Autodesk Inventor part; units mm, degrees
ref_plane "YZ Plane" through (0, 0, 0) normal (1, 0, 0) x (0, 1, 0)
ref_plane "XZ Plane" through (0, 0, 0) normal (0, 1, 0) x (-1, 0, 0)
ref_plane "XY Plane" through (0, 0, 0) normal (0, 0, 1) x (1, 0, 0)
ref_plane "Work Plane1" through (-14.5039, 0, 0) normal (0, 0, 1) x (1, 0, 0)
sketch "Sketch1" plane through (-14.5039, 0, 0) normal (0, 0, 1) x (1, 0, 0)
  line L0 (-0.3057, 380.2711) -> (-25.3057, 380.2711)
  line L1 (-25.3057, 380.2711) -> (-25.3057, 360.2711)
  line L2 (-25.3057, 360.2711) -> (-0.3057, 360.2711)
  line L3 (-0.3057, 360.2711) -> (-0.3057, 380.2711)
  arc A0 (-39.9465, 315.9933) -> (-39.9465, 424.5488) centre (-105.3057, 370.2711) ccw
  line L4 (-40.5531, 425.2711) -> (-40.5531, 315.2711) construction
  line L5 (-40.5531, 425.2711) -> (69.4469, 425.2711) construction
  line L6 (-41.4851, 315.2711) -> (-42.3392, 315.2711)
  line L7 (-41.4851, 425.2711) -> (-42.3392, 425.2711)
  arc A1 (-43.0983, 316.922) -> (-43.0983, 423.6201) centre (-105.3057, 370.2711) ccw
  arc A2 (-41.4851, 315.2711) -> (-39.9465, 315.9933) centre (-41.4851, 317.2711) ccw
  arc A3 (-39.9465, 424.5488) -> (-41.4851, 425.2711) centre (-41.4851, 423.2711) ccw
  arc A4 (-42.3392, 425.2711) -> (-43.0983, 423.6201) centre (-42.3392, 424.2711) ccw
  arc A5 (-43.0983, 316.922) -> (-42.3392, 315.2711) centre (-42.3392, 316.2711) ccw
  point P0 (14.5039, 0)
  point P1 (-44.5531, 315.2711)
  point P2 (-44.5531, 425.2711)
  point P3 (-20.938, 380.2711)
  point P4 (-20.938, 360.2711)
  dimension "d0" = 25
  dimension "d1" = 20
  dimension "d2" = 110
  dimension "d3" = 90
  dimension "d4" = 45
  dimension "d5" = 105
  dimension "d6" = 4
  dimension "d22" = 2
  dimension "d23" = 2
  dimension "d24" = 1
extrude "Extrusion1" add sketch "Sketch1" along normal blind 165 contours L3 L2 A0 L0 | A0 L2 A1 L0 | L0 A1 A4 L7 A3 A0 | A0 A2 L6 A5 A1 L2
sketch "Sketch2" plane through (-14.8095, 360.2711, 0) normal (1, 0, 0) x (0, 0, -1)
  circle A0 centre (-30, 10) radius 2.75
  circle A1 centre (-135, 10) radius 2.75
  line L0 (-165, 0) -> (-165, 20)
  line L1 (0, 0) -> (0, -44.2778)
  line L2 (-30, 10) -> (-135, 10)
  line L3 (0, -45) -> (-165, -45)
  point P0 (0, -360.2711)
  dimension "d10" = 5.5
  dimension "d11" = 5.5
  dimension "d12" = 30
  dimension "d13" = 30
  dimension "d17" = 55
extrude "Extrusion2" cut sketch "Sketch2" against normal through all
ref_plane "Work Plane2" through (-39.8095, 360.2711, 0) normal (1, 0, 0) x (0, 0, -1)
sketch "Sketch4" plane through (-39.8095, 360.2711, 0) normal (1, 0, 0) x (0, 0, -1)
  circle A0 centre (-30, 10) radius 2.75
  circle A1 centre (-30, 10) radius 5.75
  circle A2 centre (-135, 10) radius 2.75
  circle A3 centre (-135, 10) radius 5.75
  point P0 (0, -360.2711)
  dimension "d18" = 11.5
  dimension "d19" = 11.5
extrude "Extrusion3" cut sketch "Sketch4" along normal blind 20 contours A0 | A1 | A3
equation "\"d4\" = -0.5 * d1 + 0.5 * d2"
properties part number "LegSupport"
Here's how the part is built. I have some questions about the finished solid (model axes, mm). A direction names the side the tool comes from. Give positions to 0.01 mm unless a question says otherwise; leave off trailing zeros. Loops run counter-clockwise (first coordinate to the right, second up) from the corner with the lowest first, then second, coordinate; pieces in that order, holes last. Notation, with made-up numbers: M 86.5,51 L 94.5,51 A5 cw 94.5,60 Z; hole C 6,33.5 d4. An arc over 180 degrees is marked long. Return JSON: item names as keys, results as strings.
Item 1: Imagine slicing it at B-B on z = 52. List the corners of the cut face in (x, y) for me.
A:
{"outline": "M -57.6,316.92 A1 ccw -56.84,315.27 L -55.99,315.27 A2 ccw -54.45,315.99 A84.96 ccw -35.44,360.27 L -14.81,360.27 L -14.81,380.27 L -35.44,380.27 A84.96 ccw -54.45,424.55 A2 ccw -55.99,425.27 L -56.84,425.27 A1 ccw -57.6,423.62 A81.95 cw Z"}
Item 2: Imagine slicing it at D-D on x = -43. List the corners of the cut face in (y, z) for me.
A:
{"outline": "M 333.96,0 L 341.7,0 L 341.7,165 L 333.96,165 Z; M 398.84,0 L 406.58,0 L 406.58,165 L 398.84,165 Z"}
Item 3: Imagine slicing it at C-C on x = -33.5. List the corners of the cut face in (y, z) for me, then the cut area to 3 significant figures.
A:
{"outline": "M 360.27,0 L 380.27,0 L 380.27,165 L 360.27,165 Z; hole C 370.27,30 d11.5; hole C 370.27,135 d11.5", "area": "3,090 mm^2"}
Item 4: Imagine slicing it at A-A on z = 135. List the corners of the cut face in (x, y) for me, then the cut area to 3 significant figures.
A:
{"outline": "M -57.6,316.92 A1 ccw -56.84,315.27 L -55.99,315.27 A2 ccw -54.45,315.99 A84.96 ccw -35.44,360.27 L -14.81,360.27 L -14.81,367.52 L -19.81,367.52 L -19.81,364.52 L -38.06,364.52 A81.95 cw Z; M -57.6,423.62 A81.95 cw -38.06,376.02 L -19.81,376.02 L -19.81,373.02 L -14.81,373.02 L -14.81,380.27 L -35.44,380.27 A84.96 ccw -54.45,424.55 A2 ccw -55.99,425.27 L -56.84,425.27 A1 ccw Z", "area": "528 mm^2"}
Item 5: Thinking about a two-plate mould opening in Z: for faces 1 (the flat face through (-33, 371, 0)), 2 (the cylindrical face through (-41.877, 404.1, 81.345)), 3 (the cylindrical face through (-17.275, 367.586, 30.596)), which applies, released by +Z, released by -Z, zero draft, split by the parting line, or undercut?
A:
{"face 1": "released by -Z", "face 2": "zero draft", "face 3": "undercut"}
Item 6: I'm going to push flat-ended pins straight in: pin 1 Ø12 at (y, z) = (348, 106.5) entering from -X; pin 2 Ø18.5 at (y, z) = (370.27, 135) entering from -X; pin 3 Ø4 at (x, y) = (-48, 338) entering from +Z; pin 4 Ø6.5 at (y, z) = (370.27, 30) entering from -X. Where does each tip first touch, or does it pass through?
A:
{"pin 1": "stops at x = -42.89", "pin 2": "stops at x = -38.38", "pin 3": "passes through", "pin 4": "stops at x = -19.81"}
Item 7: Please list where these lines run through material, in increasing order: line 1 (Y direction, x = -30, z = 30); line 2 (Y direction, x = -18, z = 135); line 3 (Y direction, x = -21.5, z = 103.5).
A:
{"line 1": "y = 360.27 to 364.52, 376.02 to 380.27", "line 2": "y = 360.27 to 367.52, 373.02 to 380.27", "line 3": "y = 360.27 to 380.27"}
Item 8: On a 3-axis mill with a long thin cutter (end or side, diameter ignored), from which of +Z, -Z, +X, -X, +Y, -Y can I reach the whole of each face in a straight line? I mean faces 4 (the flat face through (-25, 360.271, 81)), 5 (the flat face through (-25, 380.271, 81)), 6 (the flat face through (-19.81, 369, 33)). Say none if no direction works.
A:
{"face 4": "+Z, -Z, +X, -Y", "face 5": "+Z, -Z, +X, +Y", "face 6": "-X"}
